For this review, take the finished solid that the model builds, in its own axes (mm). A direction names the side the tool comes from. Coordinates: 2 decimals unless noted, no trailing zeros. Loops run counter-clockwise (first coordinate to the right, second up) from the corner with the lowest first, then second, coordinate; pieces in that order, holes last. Notation, with made-up numbers: (25.25, 78) - (61.25, 78) arc R26 ccw to (61.25, 92) - close; hole circle Ø9 at (-14.75, 15.5). An arc over 180 degrees is marked (long way). Answer as a JSON object with one key per item and string values. Group by question number.
Item 1: We need section B-B (y = -7.5). Give the boundary of the cut face in (x, z), then the cut area to 3 significant figures.
Item 2: Tool access review of faces 1 (the flat face through (-22, 0, 38.1)), 2 (the cylindrical face through (25.96, 15.21, -43.14)), 3 (the flat face through (17, 19, -45.72)): name each direction out of +Z, -Z, +X, -X, +Y, -Y from which nothing blocks a thin tool from reaching the whole face with its end or side.
Item 3: We need section C-C (z = -3). Give the boundary of the cut face in (x, y) (1 decimal), then the cut area to 3 significant figures.
Item 4: Mouldability with a two-part tool opening along Y and no side actions: class faces 4 (the flat face through (6, -19, 50.8)), 5 (the cylindrical face through (-5.506, -24.796, 5.72)), 6 (the cylindrical face through (-9.73, -10.23, 23.67)) as released by +Y, released by -Y, zero draft, split by the parting line, or undercut.
Item 5: To check wall thickness, follow line 1 (X direction, y = 0.5, z = 28.5); line 2 (Z direction, x = 16.5, y = 7.5); line 3 (X direction, y = -19.5, z = -44). State the ranges of each line that lie inside material, in increasing order.
Item 6: We need section D-D (y = 7). Give the boundary of the cut face in (x, z), then the cut area to 3 significant figures.
Item 7: We need section A-A (x = 0). State how many separate pieces and enclosed holes the cut face has, then the cut area to 3 significant figures.
Item 8: Clearance check with flat-ended pins moving along their axes: pin 1 (4 mm diameter, centred on y = -11, z = -27.5, fed in from +X); pin 2 (25 mm diameter, centred on x = 4, y = -4.5, fed in from +Z); pin 3 (6 mm diameter, centred on y = 14.5, z = -6, fed in from -X); pin 4 (1.9 mm diameter, centred on x = -10.78, y = -10.78, fed in from +Z). State where each tip first meets the part, or that it passes through.
from build123d import *

# Parameters (mm, degrees)
SKETCH1_R           = 31.75
BOSS_EXTRUDE1_DEPTH = 50.8
SKETCH2_R           = 31.75
SKETCH2_R_2         = 25.0825
CUT_EXTRUDE1_DEPTH  = 5.08
SKETCH3_R           = 22.5425
CUT_EXTRUDE2_DEPTH  = 71.247
SKETCH4_R           = 31.75
SKETCH4_R_2         = 25.4
CUT_EXTRUDE3_DEPTH  = 91.44
SKETCH5_R           = 19.05
CUT_EXTRUDE4_DEPTH  = 24.003
SKETCH6_R           = 9.6266
CUT_EXTRUDE5_DEPTH  = 78.597
SKETCH8_R           = 1.524
CUT_EXTRUDE6_DEPTH  = 11.16
CIRPATTERN1_COUNT   = 6
SKETCH9_R           = 1.1811
CUT_EXTRUDE7_DEPTH  = 12.7
CIRPATTERN2_COUNT   = 4
SKETCH10_R          = 11.303
CUT_EXTRUDE8_DEPTH  = 1.397
SKETCH11_R          = 1.1811
CUT_EXTRUDE9_DEPTH  = 78.597
CIRPATTERN3_COUNT   = 4


with BuildPart() as part:
    # Sketch1 → Boss-Extrude1 (new body, symmetric)
    with BuildSketch(Plane.XY):
        Circle(SKETCH1_R)
    extrude(amount=BOSS_EXTRUDE1_DEPTH, both=True)

    # Sketch2 → Cut-Extrude1 (cut)
    with BuildSketch(Plane(origin=(0, 0, -50.8), x_dir=(-1, 0, 0), z_dir=(0, 0, -1))):
        Circle(SKETCH2_R)
        Circle(SKETCH2_R_2, mode=Mode.SUBTRACT)
    extrude(amount=-CUT_EXTRUDE1_DEPTH, mode=Mode.SUBTRACT)

    # Sketch3 → Cut-Extrude2 (cut)
    with BuildSketch(Plane(origin=(0, 0, -50.8), x_dir=(-1, 0, 0), z_dir=(0, 0, -1))):
        Circle(SKETCH3_R)
    extrude(amount=-CUT_EXTRUDE2_DEPTH, mode=Mode.SUBTRACT)

    # Sketch4 → Cut-Extrude3 (cut)
    with BuildSketch(Plane.XY.offset(50.8)):
        Circle(SKETCH4_R)
        Circle(SKETCH4_R_2, mode=Mode.SUBTRACT)
    extrude(amount=-CUT_EXTRUDE3_DEPTH, mode=Mode.SUBTRACT)

    # Sketch5 → Cut-Extrude4 (cut)
    with BuildSketch(Plane.XY.offset(50.8)):
        Circle(SKETCH5_R)
    extrude(amount=-CUT_EXTRUDE4_DEPTH, mode=Mode.SUBTRACT)

    # Sketch6 → Cut-Extrude5 (cut, through all)
    with BuildSketch(Plane.XY.offset(26.797)):
        Circle(SKETCH6_R)
    extrude(amount=-CUT_EXTRUDE5_DEPTH, mode=Mode.SUBTRACT)

    # Sketch8 → Cut-Extrude6 (cut, through all)
    with BuildSketch(Plane.XY.offset(-40.64)):
        with Locations((0, 28.575)):
            Circle(SKETCH8_R)
    cut_extrude6 = extrude(amount=-CUT_EXTRUDE6_DEPTH, mode=Mode.SUBTRACT)

    # CirPattern1: Cut-Extrude6 ×6 about axis
    cirpattern1_axis = Axis((0, 0, 0), (0, 0, 1))
    for i in range(1, CIRPATTERN1_COUNT):
        add(cut_extrude6.rotate(cirpattern1_axis, i * 360 / CIRPATTERN1_COUNT), mode=Mode.SUBTRACT)

    # Sketch9 → Cut-Extrude7 (cut)
    with BuildSketch(Plane.XY.offset(50.8)):
        with Locations((0, 22.225)):
            Circle(SKETCH9_R)
    cut_extrude7 = extrude(amount=-CUT_EXTRUDE7_DEPTH, mode=Mode.SUBTRACT)

    # CirPattern2: Cut-Extrude7 ×4 about axis
    cirpattern2_axis = Axis((0, 0, 0), (0, 0, 1))
    for i in range(1, CIRPATTERN2_COUNT):
        add(cut_extrude7.rotate(cirpattern2_axis, i * 360 / CIRPATTERN2_COUNT), mode=Mode.SUBTRACT)

    # Sketch10 → Cut-Extrude8 (cut)
    with BuildSketch(Plane.XY.offset(26.797)):
        Circle(SKETCH10_R)
    extrude(amount=-CUT_EXTRUDE8_DEPTH, mode=Mode.SUBTRACT)

    # Sketch11 → Cut-Extrude9 (cut, through all)
    with BuildSketch(Plane.XY.offset(26.797)):
        with Locations((-10.776307345, 10.776307345)):
            Circle(SKETCH11_R)
    cut_extrude9 = extrude(amount=-CUT_EXTRUDE9_DEPTH, mode=Mode.SUBTRACT)

    # CirPattern3: Cut-Extrude9 ×4 about axis
    cirpattern3_axis = Axis((0, 0, 0), (0, 0, 1))
    for i in range(1, CIRPATTERN3_COUNT):
        add(cut_extrude9.rotate(cirpattern3_axis, i * 360 / CIRPATTERN3_COUNT), mode=Mode.SUBTRACT)


solid = part.part
Check sheet entries:
{
 "1": {"outline": "(-30.85, -45.72) - (-23.93, -45.72) - (-23.93, -50.8) - (-21.26, -50.8) - (-21.26, 20.45) - (-6.04, 20.45) - (-6.04, 25.4) - (-8.46, 25.4) - (-8.46, 26.8) - (-17.51, 26.8) - (-17.51, 50.8) - (-24.27, 50.8) - (-24.27, -40.64) - (-30.85, -40.64) - close; (6.04, 20.45) - (21.26, 20.45) - (21.26, -50.8) - (23.93, -50.8) - (23.93, -45.72) - (30.85, -45.72) - (30.85, -40.64) - (24.27, -40.64) - (24.27, 50.8) - (17.51, 50.8) - (17.51, 26.8) - (8.46, 26.8) - (8.46, 25.4) - (6.04, 25.4) - close", "area": "1,040 mm2"},
 "2": {"face 1": "+Z", "face 2": "+Z, -Z", "face 3": "-Z"},
 "3": {"outline": "circle Ø50.8 at (0, 0); hole circle Ø45.1 at (0, 0)", "area": "430 mm2"},
 "4": {"face 4": "zero draft", "face 5": "split by the parting line", "face 6": "undercut"},
 "5": {"line 1": "x = -25.4 to -19.04, 19.04 to 25.4", "line 2": "z = 20.45 to 26.8", "line 3": "x = -25.06 to -11.31, 11.31 to 25.06"},
 "6": {"outline": "(-30.97, -45.72) - (-24.09, -45.72) - (-24.09, -50.8) - (-21.43, -50.8) - (-21.43, 20.45) - (-6.61, 20.45) - (-6.61, 25.4) - (-8.87, 25.4) - (-8.87, 26.8) - (-17.72, 26.8) - (-17.72, 50.8) - (-24.42, 50.8) - (-24.42, -40.64) - (-30.97, -40.64) - close; (6.61, 20.45) - (21.43, 20.45) - (21.43, -50.8) - (24.09, -50.8) - (24.09, -45.72) - (30.97, -45.72) - (30.97, -40.64) - (24.42, -40.64) - (24.42, 50.8) - (17.72, 50.8) - (17.72, 26.8) - (8.87, 26.8) - (8.87, 25.4) - (6.61, 25.4) - close", "area": "1,030 mm2"},
 "7": {"separate pieces": "4", "enclosed holes": "0", "area": "878 mm2"},
 "8": {"pin 1": "stops at x = 23.75", "pin 2": "stops at z = 26.8", "pin 3": "stops at x = -22.65", "pin 4": "passes through"}
}
